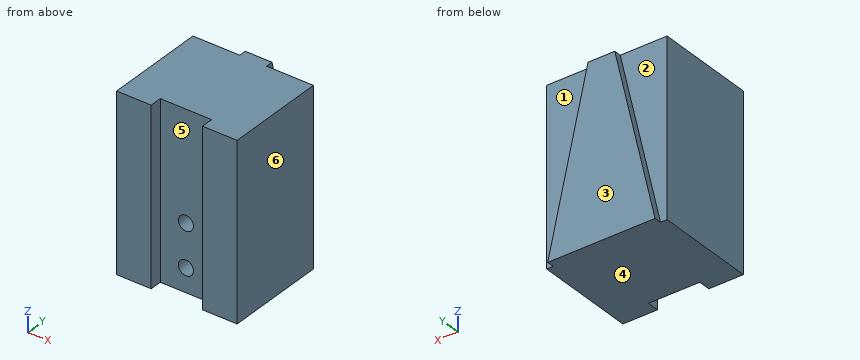
```python
from build123d import *

# Parameters (mm, degrees)
F1_DEPTH = 92.075
F3_D     = 7.9375
F3_DEPTH = 23.7998
F3_TIP   = 2.3846655818
F5_DEPTH = 3.81


with BuildPart() as f1:
    # F0 (on Top) → F1 (new body)
    with BuildSketch(Plane.XY):
        Polygon((-31.75, 57.15), (-31.75, 0), (-13.5255, 0), (-13.5255, 6.35), (13.5255, 6.35), (13.5255, 0), (31.75, 0), (31.75, 57.15), align=None)
    extrude(amount=F1_DEPTH)

    # F3
    with Locations(Plane.XZ.offset(-6.35)):
        with Locations((0, 34.8742), (0, 12.4714)):
            Hole(F3_D / 2, depth=F3_DEPTH)
            with Locations((0, 0, -(F3_DEPTH + F3_TIP / 2))):  # 118° drill point
                Cone(0, F3_D / 2, F3_TIP, mode=Mode.SUBTRACT)

    # F4 (on face) → F5 (cut)
    with BuildSketch(Plane(origin=(0, 57.15, 0), x_dir=(-1, 0, 0), z_dir=(0, 1, 0))):
        Polygon((-31.75, 0), (-28.3056886979, 0), (-7.0485, 92.075), (-31.75, 92.075), align=None)
        Polygon((7.0485, 92.075), (28.3056886979, 0), (31.75, 0), (31.75, 92.075), align=None)
    extrude(amount=-F5_DEPTH, mode=Mode.SUBTRACT)


solid = f1.part
```
Verification items for the finished model (mm, model axes). Face numbers are marked on the shaded views. A direction names the side the tool comes from. Coordinates: 2 decimals unless noted, no trailing zeros. Write each loop counter-clockwise with the first axis right and the second up, starting at its lowest first coordinate (ties: lowest second). Pieces come first, ordered by that corner, then holes. Notation, with made-up numbers: (67, 51.25) - (119, 51.25) arc R23 ccw to (119, 68.25) - close; hole circle Ø2 at (18, -36.5). An arc over 180 degrees is marked (long way). One line per question, with ' | ' between items. Start each with the question number.
1. Material ranges on line 1 along Z through (x, y) = (0, 21.5) (3 decimals); line 2 along Z through (x, y) = (1, 22) (1 decimal); line 3 along Y through (x, z) = (20, 57), recorded low to high.
2. Access from +Z, -Z, +X, -X, +Y, -Y to the whole of each face (thin tool, end or side, straight path). Record for the marked faces 1, 2 and 3.
3. Gauge pin test, flat ends, axial feed: P1, Ø12.5, axis at x = 0, z = 12.47, coming from the -Y side; P2, Ø13.5, axis at x = 2, z = 63, coming from the -Y side. Record the tip position at first contact, or that the pin passes through.
4. Section check D-D (z = 54). Enter the section's corners in (x, y).
5. Section check B-B (y = 28). Count the separate pieces of the cut face and the enclosed holes in it, plus the area to 3 significant figures.
6. Draft check along X on the marked faces 4, 5 and 6. Enter one of: released by +X, released by -X, zero draft, split by the parting line, or undercut.
7. Section check C-C (x = 11.5). Enter the section's corners in (y, z) (3 decimals).
8. Section check A-A (z = 41). Enter the section's corners in (x, y), plus the area to 3 significant figures.
Computed values:
1) line 1: 0 to 8.503, 16.44 to 30.905, 38.843 to 92.075 | line 2: 0 to 8.6, 16.3 to 31, 38.7 to 92.1 | line 3: 0 to 53.34
2) face 1: +Z, +X, +Y | face 2: +Z, -X, +Y | face 3: +Z, -Z, +X, -X, +Y
3) P1: y = 6.35 | P2: y = 6.35
4) outline: (-31.75, 0) - (-13.53, 0) - (-13.53, 6.35) - (13.53, 6.35) - (13.53, 0) - (31.75, 0) - (31.75, 53.34) - (15.84, 53.34) - (15.84, 57.15) - (-15.84, 57.15) - (-15.84, 53.34) - (-31.75, 53.34) - close
5) separate pieces: 1 | enclosed holes: 2 | area: 5,750 mm²
6) face 4: zero draft | face 5: undercut | face 6: released by +X
7) outline: (6.35, 0) - (57.15, 0) - (57.15, 72.793) - (53.34, 72.793) - (53.34, 92.075) - (6.35, 92.075) - close
8) outline: (-31.75, 0) - (-13.53, 0) - (-13.53, 6.35) - (13.53, 6.35) - (13.53, 0) - (31.75, 0) - (31.75, 53.34) - (18.84, 53.34) - (18.84, 57.15) - (-18.84, 57.15) - (-18.84, 53.34) - (-31.75, 53.34) - close | area: 3,360 mm²
